The model under review builds one solid part; all positions refer to its coordinate system, in mm. Face numbers are marked on the shaded views. A direction names the side the tool comes from. Coordinates: 2 decimals unless noted, no trailing zeros. Write each loop counter-clockwise with the first axis right and the second up, starting at its lowest first coordinate (ties: lowest second). Pieces come first, ordered by that corner, then holes. Notation, with made-up numbers: (18, 43.25) - (53, 43.25) arc R25 cw to (53, 79.25) - close; hole circle Ø10 at (-14.5, -25.5). An arc over 180 degrees is marked (long way). Use one line per item in the form item = value. Start each with the question number.
```python
from build123d import *

# Parameters (mm, degrees)
SKETCH1_W           = 50
SKETCH1_H           = 40
BOSS_EXTRUDE1_DEPTH = 32
BOSS_EXTRUDE2_DEPTH = 38
BOSS_EXTRUDE3_START = 6
BOSS_EXTRUDE3_DEPTH = 6
SKETCH2_W           = 40
SKETCH2_H           = 30
SKETCH2_H_2         = 11
CUT_EXTRUDE1_DEPTH  = 22
BOSS_EXTRUDE5_DEPTH = 3
BOSS_EXTRUDE6_START = 3
BOSS_EXTRUDE6_DEPTH = 3
CUT_EXTRUDE2_DEPTH  = 5


with BuildPart() as part:
    # Sketch1 → Boss-Extrude1 (new body)
    with BuildSketch(Plane.XY):
        Rectangle(SKETCH1_W, SKETCH1_H)
    extrude(amount=-BOSS_EXTRUDE1_DEPTH)

    # Sketch1_3 → Boss-Extrude2 (add)
    with BuildSketch(Plane.XY):
        with BuildLine():
            Line((-3, -20), (-25, -20))
            Line((-25, -20), (-25, -52))
            ThreePointArc((-25, -52), (-14, -41), (-3, -52))
            Line((-3, -52), (-3, -20))
        make_face()
        with BuildLine():
            ThreePointArc((-3, -52), (-14, -41), (-25, -52))
            Line((-25, -52), (-3, -52))
        make_face()
        with BuildLine():
            Line((-3, -52), (-25, -52))
            ThreePointArc((-25, -52), (-14, -63), (-3, -52))
        make_face()
    extrude(amount=-BOSS_EXTRUDE2_DEPTH)

    # Sketch1_4 → Boss-Extrude3 (add)
    with BuildSketch(Plane.XY.offset(BOSS_EXTRUDE3_START)):
        with BuildLine():
            Line((-3, -20), (-25, -20))
            Line((-25, -20), (-25, -52))
            ThreePointArc((-25, -52), (-14, -41), (-3, -52))
            Line((-3, -52), (-3, -20))
        make_face()
        with BuildLine():
            ThreePointArc((-3, -52), (-14, -41), (-25, -52))
            Line((-25, -52), (-3, -52))
        make_face()
        with BuildLine():
            Line((-3, -52), (-25, -52))
            ThreePointArc((-25, -52), (-14, -63), (-3, -52))
        make_face()
    extrude(amount=-BOSS_EXTRUDE3_DEPTH)

    # Sketch2 → Cut-Extrude1 (cut)
    with BuildSketch(Plane.ZY.offset(25)):
        with Locations((-16, -37)):
            Rectangle(SKETCH2_W, SKETCH2_H)
        with Locations((-16, -57.5)):
            Rectangle(SKETCH2_W, SKETCH2_H_2)
    extrude(amount=-CUT_EXTRUDE1_DEPTH, mode=Mode.SUBTRACT)

    # Sketch3 → Boss-Extrude5 (add)
    with BuildSketch(Plane(origin=(0, 0, 4), x_dir=(-1, 0, 0), z_dir=(0, 0, -1))):
        with BuildLine():
            ThreePointArc((3, -52), (14, -63), (25, -52))
            Line((25, -52), (3, -52))
        make_face()
        with BuildLine():
            Line((3, -52), (25, -52))
            ThreePointArc((25, -52), (14, -41), (3, -52))
        make_face()
        with BuildLine():
            Line((25, -52), (3, -52))
            ThreePointArc((3, -52), (14, -63), (25, -52))
        make_face()
    extrude(amount=BOSS_EXTRUDE5_DEPTH)

    # Sketch4 → Boss-Extrude6 (add)
    with BuildSketch(Plane.XY.offset(-36).offset(BOSS_EXTRUDE6_START)):
        with BuildLine():
            ThreePointArc((-3, -52), (-14, -41), (-25, -52))
            Line((-25, -52), (-3, -52))
        make_face()
        with BuildLine():
            Line((-3, -52), (-25, -52))
            ThreePointArc((-25, -52), (-14, -63), (-3, -52))
        make_face()
        with BuildLine():
            Line((-25, -52), (-3, -52))
            ThreePointArc((-3, -52), (-14, -63), (-25, -52))
        make_face()
    extrude(amount=-BOSS_EXTRUDE6_DEPTH)

    # Sketch13 → Cut-Extrude2 (cut)
    with BuildSketch(Plane(origin=(0, 20, 0), x_dir=(1, 0, 0), z_dir=(0, 1, 0))):
        with BuildLine():
            ThreePointArc((24, 16), (14, 26), (4, 16))
            Line((4, 16), (24, 16))
        make_face()
        with BuildLine():
            Line((24, 16), (4, 16))
            ThreePointArc((4, 16), (14, 6), (24, 16))
        make_face()
    extrude(amount=-CUT_EXTRUDE2_DEPTH, mode=Mode.SUBTRACT)


solid = part.part
```
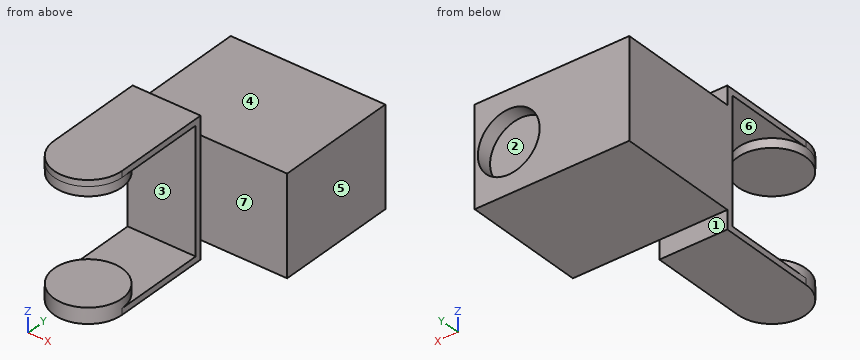
1. For the marked faces 1, 2, 3 and 4, list the 3-axis set-ups (+Z, -Z, +X, -X, +Y, -Y) from which the entire face can be reached by the end or side of a thin tool; tool diameter is ignored.
2. For P1, Ø12, axis at x = -18, y = 3.5, coming from the -Z side; P2, Ø17.5, axis at x = -13.5, z = -12.5, coming from the -Y side; P3, Ø1, axis at x = -11, y = -0.5, coming from the +Z side, all flat-tipped, find the tip position at first contact; note any pin that passes through.
3. Take a section at C-C (y = -53). State the section outline as (x, z) points.
4. Take a section at B-B (x = 14). State the section outline as (y, z) points, plus the area to 3 significant figures.
5. For L1, parallel to Z at x = -23, y = -32; L2, parallel to Z at x = 14, y = 16; L3, parallel to Z at x = 20, y = 5, list the stretches that pass through material, from the lowest coordinate up.
6. Take a section at D-D (x = -14). State the section outline as (y, z) points.
7. The part is to be moulded in two halves that separate along Y. For the marked faces 5, 6 and 7, say which applies: released by +Y, released by -Y, zero draft, split by the parting line, or undercut.
8. Take a section at A-A (z = -16). State the section outline as (x, y) points.
Returned:
q1.face_1 = -Z, +X, -X, +Y
q1.face_2 = +Y
q1.face_3 = +X, -X
q1.face_4 = +Z, +X, -X, +Y
q2.P1 = -32
q2.P2 = -22
q2.P3 = 0
q3.outline = (-24.95, -38) - (-3.05, -38) - (-3.05, -33) - (-24.95, -33) - close; (-24.95, 1) - (-3.05, 1) - (-3.05, 6) - (-24.95, 6) - close
q4.outline = (-20, -32) - (20, -32) - (20, -26) - (15, -26) - (15, -6) - (20, -6) - (20, 0) - (-20, 0) - close
q4.area = 1,180 mm²
q5.L1 = -38 to -36, 4 to 6
q5.L2 = -32 to -26, -6 to 0
q5.L3 = -32 to 0
q6.outline = (-63, -38) - (-20, -38) - (-20, -32) - (20, -32) - (20, 0) - (-20, 0) - (-20, 6) - (-63, 6) - (-63, 1) - (-41, 1) - (-41, 4) - (-22, 4) - (-22, -36) - (-41, -36) - (-41, -33) - (-63, -33) - close
q7.face_5 = zero draft
q7.face_6 = undercut
q7.face_7 = released by -Y
q8.outline = (-25, -22) - (-3, -22) - (-3, -20) - (25, -20) - (25, 20) - (24, 20) - (24, 15) - (4, 15) - (4, 20) - (-25, 20) - close
